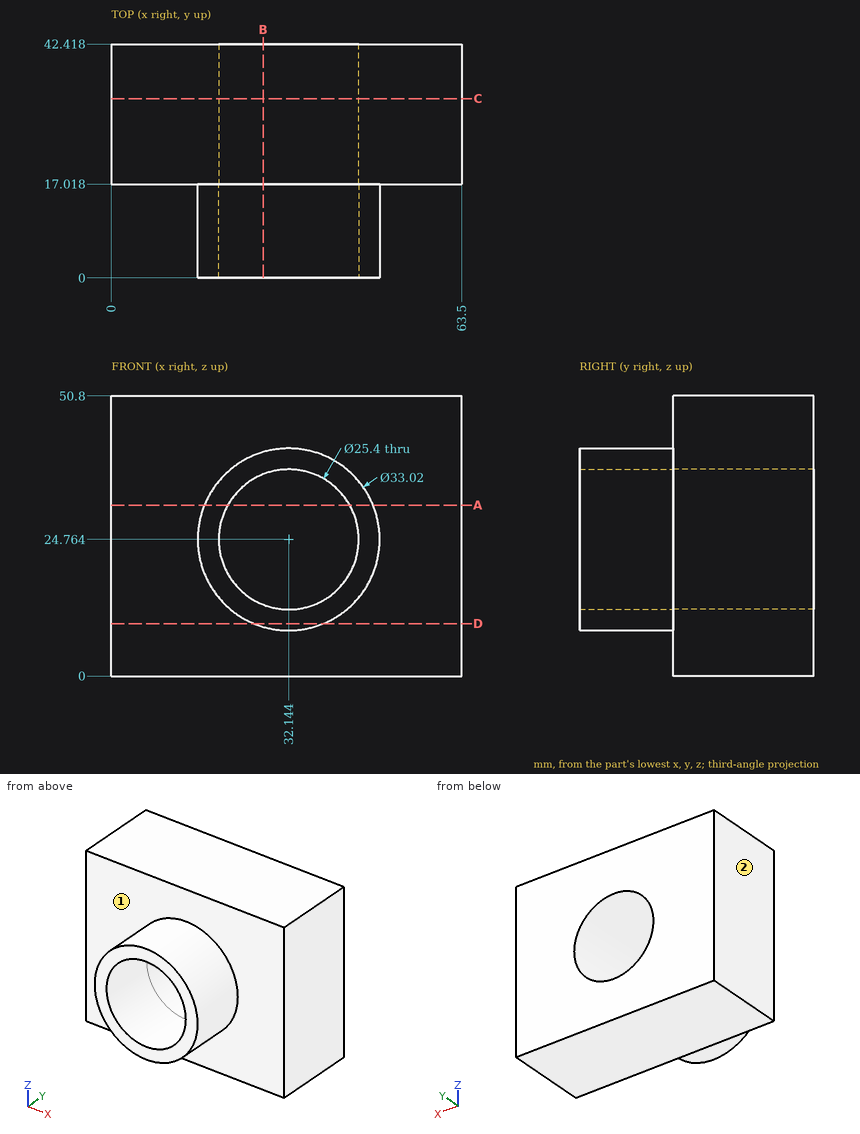
Verification items for this drawing (mm, ordinates from the low corner). A direction names the side the tool comes from. Coordinates: 2 decimals unless noted, no trailing zeros. Order: outer loops, then holes, each group sorted by start corner. A loop starts at its lowest first (then second) coordinate and runs counter-clockwise, first axis right, second up. Notation, with made-up numbers: (-31.75, 26) - (17.25, 26) arc R28 cw to (17.25, 52) - close; hole circle Ø8 at (38, 34). An arc over 180 degrees is marked (long way). Answer in a Markdown table with one row per item. Add a question column.
1. Section check A-A (z = 31). Enter the section's corners in (x, y).
2. Section check B-B (x = 27.5). Enter the section's corners in (y, z).
3. Section check D-D (z = 9.5). Enter the section's corners in (x, y), plus the area to 3 significant figures.
4. Material ranges on L1, parallel to Y at x = 7, z = 27.5; L2, parallel to Z at x = 29, y = 30.5; L3, parallel to Z at x = 25.5, y = 27.5, recorded low to high. Write a range as [from, to].
5. Section check C-C (y = 32.5). Enter the section's corners in (x, z), plus the area to 3 significant figures.
6. Access from +Z, -Z, +X, -X, +Y, -Y to the whole of each face (thin tool, end or side, straight path). Record for the marked faces 1 and 2.
7. Gauge pin test, flat ends, axial feed: pin 1 Ø2 at (y, z) = (5, 21) entering from +X; pin 2 Ø1.5 at (x, y) = (23.5, 11.5) entering from +Z; pin 3 Ø23 at (x, z) = (32.14, 24.76) entering from -Y. Record the tip position at first contact, or that the pin passes through.
Data:
| question | item | result |
|---|---|---|
| 1 | outline | (0, 17.02) - (16.86, 17.02) - (16.86, 0) - (21.08, 0) - (21.08, 42.42) - (0, 42.42) - close; (43.21, 0) - (47.43, 0) - (47.43, 17.02) - (63.5, 17.02) - (63.5, 42.42) - (43.21, 42.42) - close |
| 2 | outline | (0, 8.92) - (17.02, 8.92) - (17.02, 0) - (42.42, 0) - (42.42, 12.94) - (0, 12.94) - close; (0, 36.58) - (42.42, 36.58) - (42.42, 50.8) - (17.02, 50.8) - (17.02, 40.61) - (0, 40.61) - close |
| 3 | outline | (0, 17.02) - (25.85, 17.02) - (25.85, 0) - (38.44, 0) - (38.44, 17.02) - (63.5, 17.02) - (63.5, 42.42) - (0, 42.42) - close |
| 3 | area | 1,830 mm² |
| 4 | L1 | y = [17.02, 42.42] |
| 4 | L2 | z = [0, 12.46], [37.07, 50.8] |
| 4 | L3 | z = [0, 13.94], [35.59, 50.8] |
| 5 | outline | (0, 0) - (63.5, 0) - (63.5, 50.8) - (0, 50.8) - close; hole circle Ø25.4 at (32.14, 24.76) |
| 5 | area | 2,720 mm² |
| 6 | face 1 | -Y |
| 6 | face 2 | +Z, -Z, -X, +Y, -Y |
| 7 | pin 1 | stops at x = 48.42 |
| 7 | pin 2 | stops at z = 39.26 |
| 7 | pin 3 | passes through |
